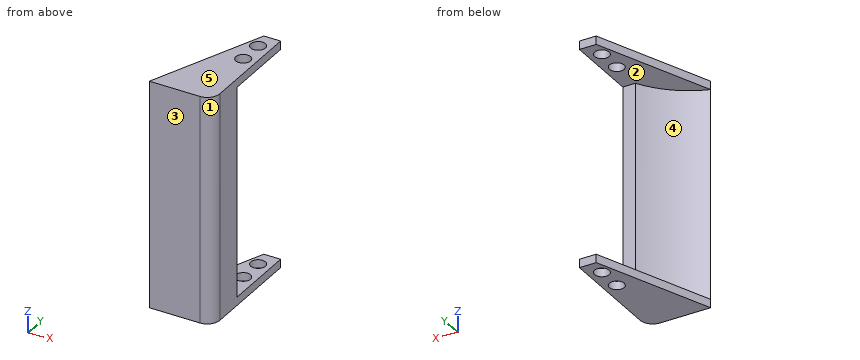
from build123d import *

# Parameters (mm, degrees)
BOSS_EXTRUDE1_DEPTH = 25
SKETCH2_R           = 1.75
BOSS_EXTRUDE2_DEPTH = 2
FILLET1_R           = 3


with BuildPart() as part:
    # Sketch1 → Boss-Extrude1 (new, symmetric)
    with BuildSketch(Plane.XY):
        with BuildLine():
            Line((0, 0), (15, 0))
            Line((15, 0), (15, 10))
            Line((15, 10), (12, 10))
            ThreePointArc((12, 10), (6.940286442, 3.871656269), (0, 0))
        make_face()
    extrude(amount=BOSS_EXTRUDE1_DEPTH, both=True)

    # Sketch2 → Boss-Extrude2 (add)
    with BuildSketch(Plane.XY.offset(25)):
        Polygon((15, 0), (15, 27.5), (11, 27.5), (0, 0), align=None)
        with Locations((12, 23.5)):
            Circle(SKETCH2_R, mode=Mode.SUBTRACT)
        with Locations((12, 17.5)):
            Circle(SKETCH2_R, mode=Mode.SUBTRACT)
    boss_extrude2 = extrude(amount=BOSS_EXTRUDE2_DEPTH)

    # Mirror1: Boss-Extrude2 across plane
    add(boss_extrude2.mirror(Plane.XY))

    # Fillet1
    fillet1_edges = [part.edges().sort_by_distance(p)[0] for p in [
        (15, 0, 0),
    ]]
    fillet(fillet1_edges, radius=FILLET1_R)


solid = part.part
Can you work these out from the model? Positions are in its coordinate system, mm. Face numbers are marked on the shaded views. A direction names the side the tool comes from. Coordinates: 2 decimals unless noted, no trailing zeros. Loops run counter-clockwise (first coordinate to the right, second up) from the corner with the lowest first, then second, coordinate; pieces in that order, holes last. Notation, with made-up numbers: M 23,20 L 47,20 A18 cw 47,55 Z; hole C 76.25,16.25 d2. An arc over 180 degrees is marked long. Return JSON: item names as keys, results as strings. Group by question number.
Item 1: I'm going to push a flat-ended pin straight in: pin 1 Ø3.5 at (x, z) = (14, 10.5) entering from +Y. Where does the tip first touch, or does it pass through?
Item 2: Imagine slicing it at C-C (x = 12.5). Please give me the cut outline in (y, z).
Item 3: Thinking about a two-plate mould opening in Z: for the marked faces 3, 4 and 5, which applies, released by +Z, released by -Z, zero draft, split by the parting line, or undercut?
Item 4: If I drill on L1, parallel to Y at x = 12, z = -25.75; L2, parallel to Z at x = 13.5, y = 16.25; L3, parallel to Y at x = 5.75, z = 22.5, over which ranges is the centre line in solid material (lowest first)? Write a range as from..to.
Item 5: Imagine slicing it at B-B (y = 13). Please give me the cut outline in (x, z), and give its area (3 significant figures).
Item 6: On a 3-axis mill with a long thin cutter (end or side, diameter ignored), from which of +Z, -Z, +X, -X, +Y, -Y can I reach the whole of each face in a straight line? I mean the marked faces 1 and 2. Say none if no direction works.
Item 7: Imagine slicing it at D-D (y = 17.5). Please give me the cut outline in (x, z).
Item 8: Imagine slicing it at A-A (y = 23.5). Please give me the cut outline in (x, z).
Verdict:
{
 "1": {"pin 1": "stops at y = 10"},
 "2": {"outline": "M 0.04,-27 L 15.82,-27 L 15.82,-25 L 10,-25 L 10,25 L 15.82,25 L 15.82,27 L 0.04,27 Z; M 19.18,-27 L 21.82,-27 L 21.82,-25 L 19.18,-25 Z; M 19.18,25 L 21.82,25 L 21.82,27 L 19.18,27 Z; M 25.18,-27 L 27.5,-27 L 27.5,-25 L 25.18,-25 Z; M 25.18,25 L 27.5,25 L 27.5,27 L 25.18,27 Z"},
 "3": {"face 3": "zero draft", "face 4": "undercut", "face 5": "released by +Z"},
 "4": {"L1": "y = 0..15.75, 19.25..21.75, 25.25..27.5", "L2": "z = -27..-25, 25..27", "L3": "y = 0..2.95"},
 "5": {"outline": "M 5.2,-27 L 15,-27 L 15,-25 L 5.2,-25 Z; M 5.2,25 L 15,25 L 15,27 L 5.2,27 Z", "area": "39.2 mm^2"},
 "6": {"face 1": "+Z, -Z, +X, -Y", "face 2": "-X, +Y"},
 "7": {"outline": "M 7,-27 L 10.25,-27 L 10.25,-25 L 7,-25 Z; M 7,25 L 10.25,25 L 10.25,27 L 7,27 Z; M 13.75,-27 L 15,-27 L 15,-25 L 13.75,-25 Z; M 13.75,25 L 15,25 L 15,27 L 13.75,27 Z"},
 "8": {"outline": "M 9.4,-27 L 10.25,-27 L 10.25,-25 L 9.4,-25 Z; M 9.4,25 L 10.25,25 L 10.25,27 L 9.4,27 Z; M 13.75,-27 L 15,-27 L 15,-25 L 13.75,-25 Z; M 13.75,25 L 15,25 L 15,27 L 13.75,27 Z"}
}
